Source: CAD feature listing. Evaluate the final solid. Frame: model axes, mm. A direction names the side the tool comes from. Give positions to 0.01 mm unless a question says otherwise; leave off trailing zeros. Order: outer loops, then holes, each group sorted by start corner. A loop starts at its lowest first (then second) coordinate and runs counter-clockwise, first axis right, second up. Notation, with made-up numbers: (-9, 75) - (42, 75) arc R7 cw to (42, 83) - close; hole circle Ø3 at (45.25, 69.5). An arc over 180 degrees is marked (long way). Use CSV: the item, a comma, the result in double quotes.
```python
from build123d import *

# Parameters (mm, degrees)
BOSS_EXTRUDE1_DEPTH = 6
SKETCH2_W           = 71
SKETCH2_H           = 25
SKETCH2_W_2         = 5
SKETCH2_H_2         = 15
SKETCH2_W_3         = 47
SKETCH2_H_3         = 57
CUT_EXTRUDE1_DEPTH  = 176.513532242


with BuildPart() as part:
    # Sketch1 → Boss-Extrude1 (new body)
    with BuildSketch(Plane(origin=(0, 0, 0), x_dir=(1, 0, 0), z_dir=(0, 1, 0))):
        Polygon((0, 135), (0, 105.585), (6, 105.585), (6, 81.195), (0, 81.195), (0, 56.805), (6, 56.805), (6, 32.415), (0, 32.415), (0, 8.025), (0, 3), (19.415, 3), (19.415, 9), (43.805, 9), (43.805, 3), (68.195, 3), (68.195, 9), (92.585, 9), (92.585, 3), (112, 3), (112, 32.415), (106, 32.415), (106, 56.805), (112, 56.805), (112, 81.195), (106, 81.195), (106, 105.585), (112, 105.585), (112, 129.975), (112, 135), (92.585, 135), (92.585, 129), (68.195, 129), (68.195, 135), (43.805, 135), (43.805, 129), (19.415, 129), (19.415, 135), align=None)
    extrude(amount=BOSS_EXTRUDE1_DEPTH)

    # Sketch2 → Cut-Extrude1 (cut, through all)
    with BuildSketch(Plane(origin=(0, 6, 0), x_dir=(1, 0, 0), z_dir=(0, 1, 0))):
        with Locations((56, 98.5)):
            Rectangle(SKETCH2_W, SKETCH2_H)
        with Locations((94, 98.5)):
            Rectangle(SKETCH2_W_2, SKETCH2_H_2)
        with Locations((56, 47.5)):
            Rectangle(SKETCH2_W_3, SKETCH2_H_3)
    extrude(amount=-CUT_EXTRUDE1_DEPTH, mode=Mode.SUBTRACT)


solid = part.part
```
Item 1: First-contact query: pin 1 (2 mm diameter, centred on x = 40.5, y = 2.5, fed in from +Z); pin 2 (1.8 mm diameter, centred on x = 32.5, y = 1.5, fed in from -Z); pin 3 (3 mm diameter, centred on y = 3, z = -42, fed in from -X). Flat tips, straight axial feed; report the tip coordinate or a pass-through.
Filled in:
pin 1,"stops at z = -9"
pin 2,"stops at z = -129"
pin 3,"stops at x = 6"
Item 2: Section D-D on y = 2.05. Count the separate pieces of the cut face and the enclosed holes in it, then the cut area to 3 significant figures.
Filled in:
separate pieces,"1"
enclosed holes,"2"
area,"9,080 mm2"
Item 3: Section C-C on z = -25.5. Return the cut outline in (x, y).
Filled in:
outline,"(0, 0) - (32.5, 0) - (32.5, 6) - (0, 6) - close; (79.5, 0) - (112, 0) - (112, 6) - (79.5, 6) - close"
Item 4: Material intervals for line 1 (Z direction, x = 51, y = 3.45); line 2 (Z direction, x = 70, y = 2.95); line 3 (X direction, y = 5, z = -100), sorted ascending. Write a range as from..to.
Filled in:
line 1,"z = -135..-111, -86..-76, -19..-3"
line 2,"z = -129..-111, -86..-76, -19..-9"
line 3,"x = 6..20.5, 96.5..106"
Item 5: Section A-A on z = -55. Return the cut outline in (x, y).
Filled in:
outline,"(6, 0) - (32.5, 0) - (32.5, 6) - (6, 6) - close; (79.5, 0) - (106, 0) - (106, 6) - (79.5, 6) - close"
Item 6: Section B-B on x = 41. Return the cut outline in (y, z).
Filled in:
outline,"(0, -129) - (6, -129) - (6, -111) - (0, -111) - close; (0, -86) - (6, -86) - (6, -76) - (0, -76) - close; (0, -19) - (6, -19) - (6, -9) - (0, -9) - close"
Item 7: Set-up query: faces 4 (the flat face through (68.195, 3, -6)), 5 (the flat face through (32, 3, -129)), 6 (the flat face through (91.5, 3, -88)), 7 (the flat face through (109, 3, -56.805)). Return all of +Z, -Z, +X, -X, +Y, -Y with unobstructed straight access to the full face (end or side cutting, diameter ignored); none if empty.
Filled in:
face 4,"+Z, +Y, -Y"
face 5,"-Z, +Y, -Y"
face 6,"+Y, -Y"
face 7,"+X, +Y, -Y"
Item 8: Mould query, pull axis X, two halves, no side actions, for faces 1 (the flat face through (112, 3, -69)), 2 (the flat face through (31, 3, -9)), 3 (the flat face through (3, 3, -32.415)). Classes: released by +X, released by -X, zero draft, split by the parting line, or undercut.
Filled in:
face 1,"released by +X"
face 2,"undercut"
face 3,"zero draft"
